Study the drawing (mm; zero at the part's minimum x, y, z) and answer. A direction names the side the tool comes from. Coordinates: 2 decimals unless noted, no trailing zeros. Loops run counter-clockwise (first coordinate to the right, second up) from the corner with the lowest first, then second, coordinate; pieces in that order, holes last. Notation, with made-up numbers: M -22.5,-22 L -17.5,-22 A16 ccw -17.5,4 Z; hole C 10.25,-2.75 d5. An arc over 180 degrees is marked long. Use one line per item in the form item = value. Start each with the question number.
1. The part is cut by section C-C (x = 5.5). Give the vertices of the cut face in (y, z) (1 decimal), plus the area to 3 significant figures.
2. Flat-ended cylindrical pins translate along their axes: pin 1 (0.9 mm diameter, centred on y = 35.5, z = 11.5, fed in from -X); pin 2 (11 mm diameter, centred on x = 29.5, y = 21, fed in from -Z); pin 3 (3 mm diameter, centred on x = 31, y = 26, fed in from +Z). Find the tip coordinate at first contact, or state that the pin passes through.
3. The part is cut by section A-A (z = 3.25). Give the vertices of the cut face in (x, y) (1 decimal), plus the area to 3 significant figures.
4. A tool of negligible diameter and unlimited length cuts with its end or side. For the marked faces 1, 2 and 3, from which of +Z, -Z, +X, -X, +Y, -Y can it reach the whole face along a straight path? Write none if from no direction.
5. The part is cut by section B-B (y = 37.5). Give the vertices of the cut face in (x, z).
6. Find the intervals of material crossed by probe 1 along Z at (x, y) = (32.5, 53.5); probe 2 along X at (y, z) = (18.5, 10.5); probe 3 along Y at (x, z) = (37, 19.25) (1 decimal), in increasing order. Write a range as [from, to].
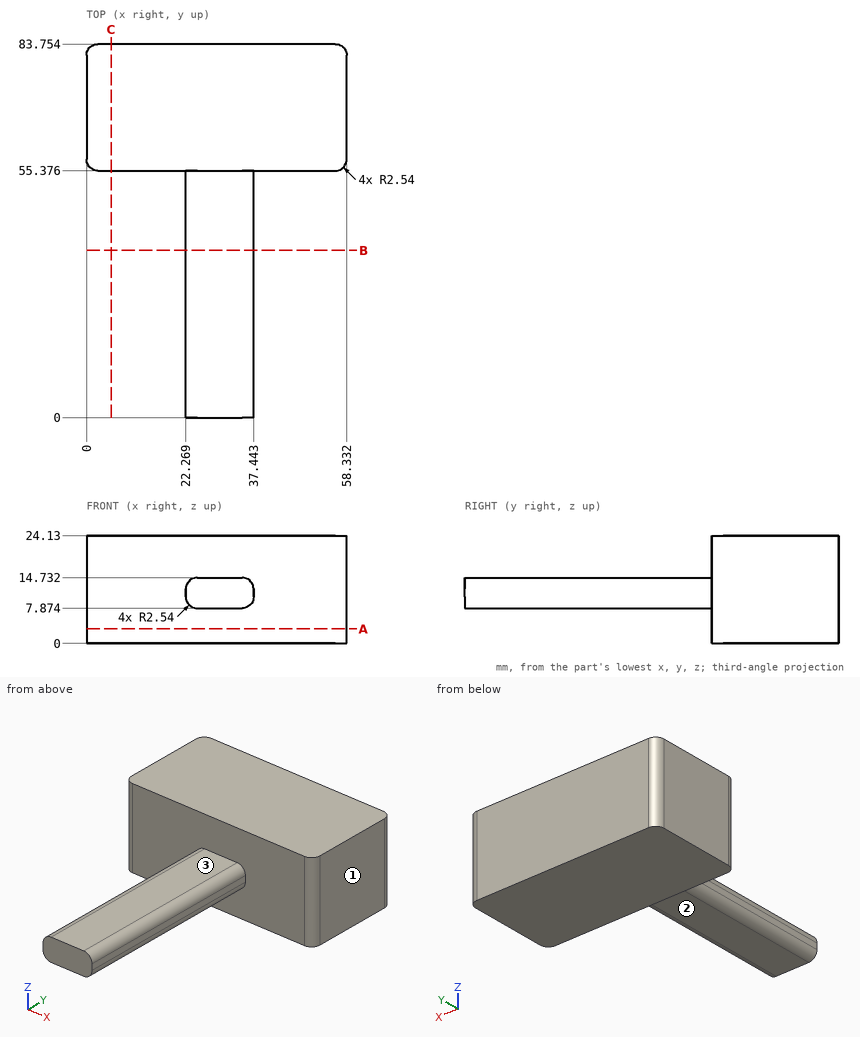
Computed values:
q1.outline = M 55.4,0 L 83.8,0 L 83.8,24.1 L 55.4,24.1 Z
q1.area = 685 mm²
q2.pin_1 = 22.27
q2.pin_2 = 7.87
q2.pin_3 = 14.73
q3.outline = M 0,57.9 A2.5 ccw 2.5,55.4 L 55.8,55.4 A2.5 ccw 58.3,57.9 L 58.3,81.2 A2.5 ccw 55.8,83.8 L 2.5,83.8 A2.5 ccw 0,81.2 Z
q3.area = 1,650 mm²
q4.face_1 = +Z, -Z, +X, +Y, -Y
q4.face_2 = -Z, +X, -X, -Y
q4.face_3 = +Z, +X, -X, -Y
q5.outline = M 22.27,10.41 A2.54 ccw 24.81,7.87 L 34.9,7.87 A2.54 ccw 37.44,10.41 L 37.44,12.19 A2.54 ccw 34.9,14.73 L 24.81,14.73 A2.54 ccw 22.27,12.19 Z
q6.probe_1 = [7.87, 14.73]
q6.probe_2 = [22.27, 37.44]
q6.probe_3 = [55.4, 83.8]
